Check sheet for the modelled part. Datum: model origin and axes. Units: mm. Round coordinates to 2 decimals unless told otherwise and drop trailing zeros. Loops run counter-clockwise (first coordinate to the right, second up) from the corner with the lowest first, then second, coordinate; pieces in that order, holes last. Notation, with made-up numbers: M 10.25,50 L 37.25,50 A17 cw 37.25,73 Z; hole C 73.25,8.25 d2. An arc over 180 degrees is marked long. One line per question, with ' | ' between items. Start each with the question number.
(1) Draft check along Y on faces 1 (the face through (55.076, 154.307, -0.986)), 2 (the face through (27, 58, 0)). Enter one of: +Y half, -Y half, draft (parallel to the pull), parting line (faces both ways), or undercut.
(2) Section check A-A (x = -23). Record the boundary of the cut face in (y, z), and give its area (3 significant figures).
(3) Section check C-C (y = 34). Record the boundary of the cut face in (x, z), and give its area (3 significant figures).
(4) Thickness scan on probe 1 along X at (y, z) = (214.3, -1.4); probe 2 along X at (y, z) = (191.85, -0.95); probe 3 along Y at (x, z) = (-31.35, -1.35). Record the ranges inside material, lowest first. Write a range as [from, to].
(5) Section check B-B (z = -0.85). Count the separate pieces of the cut face and the enclosed holes in it, and give its area (3 significant figures).
(6) Go/stop test with a flat-tipped pin: P1, Ø2, axis at x = 16.5, y = 27, coming from the +Z side. Record where the tip stops, or that it passes through.
```python
from build123d import *

# Parameters (mm, degrees)
SKETCH1_R           = 1.6
SKETCH1_R_2         = 20
SKETCH1_R_3         = 1.25
BOSS_EXTRUDE1_DEPTH = 2


with BuildPart() as part:
    # Sketch1 → Boss-Extrude1 (new body)
    with BuildSketch(Plane(origin=(0, 0, 0), x_dir=(0, 1, 0), z_dir=(0, 0, 1))):
        Polygon((-98, 35), (-98, -90), (219.3, -90), (219.3, 35), (106.85, 35), (106.85, 6.35), (-57.15, 6.35), (-57.15, 35), align=None)
        with Locations(Location((205.3, 7.8, 0), (0, 0, 270))):
            Circle(SKETCH1_R, mode=Mode.SUBTRACT)
        with Locations(Location((-92.5, 8, 0), (0, 0, 270))):
            Circle(SKETCH1_R, mode=Mode.SUBTRACT)
        with Locations(Location((-93, 28, 0), (0, 0, 270))):
            Circle(SKETCH1_R, mode=Mode.SUBTRACT)
        with Locations(Location((114.3, 0, 0), (0, 0, 270))):
            Circle(SKETCH1_R, mode=Mode.SUBTRACT)
        with Locations(Location((-93, -83, 0), (0, 0, 270))):
            Circle(SKETCH1_R, mode=Mode.SUBTRACT)
        with Locations(Location((-86.5, -73, 0), (0, 0, 270))):
            Circle(SKETCH1_R, mode=Mode.SUBTRACT)
        with Locations(Location((64.3, -83, 0), (0, 0, 270))):
            Circle(SKETCH1_R, mode=Mode.SUBTRACT)
        with Locations(Location((75.7, -78, 0), (0, 0, 270))):
            Circle(SKETCH1_R, mode=Mode.SUBTRACT)
        with Locations(Location((214.3, -83, 0), (0, 0, 270))):
            Circle(SKETCH1_R, mode=Mode.SUBTRACT)
        with Locations(Location((208.3, -65, 0), (0, 0, 270))):
            Circle(SKETCH1_R, mode=Mode.SUBTRACT)
        with Locations(Location((181.3, -56, 0), (0, 0, 270))):
            Circle(SKETCH1_R, mode=Mode.SUBTRACT)
        with Locations(Location((148.3, -36, 0), (0, 0, 270))):
            Circle(SKETCH1_R_2, mode=Mode.SUBTRACT)
        with Locations(Location((0, 0, 0), (0, 0, 270))):
            Circle(SKETCH1_R, mode=Mode.SUBTRACT)
        with Locations(Location((104.8, -18, 0), (0, 0, 270))):
            Circle(SKETCH1_R, mode=Mode.SUBTRACT)
        with Locations(Location((191.85, 31.35, 0), (0, 0, 270))):
            Circle(SKETCH1_R_3, mode=Mode.SUBTRACT)
        with Locations(Location((121.85, 11.35, 0), (0, 0, 270))):
            Circle(SKETCH1_R_3, mode=Mode.SUBTRACT)
        with Locations(Location((111.3, 28, 0), (0, 0, 270))):
            Circle(SKETCH1_R, mode=Mode.SUBTRACT)
        with Locations(Location((121.85, 31.35, 0), (0, 0, 270))):
            Circle(SKETCH1_R_3, mode=Mode.SUBTRACT)
        with Locations(Location((191.85, 11.35, 0), (0, 0, 270))):
            Circle(SKETCH1_R_3, mode=Mode.SUBTRACT)
        with Locations(Location((214.3, 28, 0), (0, 0, 270))):
            Circle(SKETCH1_R, mode=Mode.SUBTRACT)
    extrude(amount=-BOSS_EXTRUDE1_DEPTH)


solid = part.part
```
The answers:
1) face 1: undercut | face 2: draft
2) outline: M -98,-2 L -57.15,-2 L -57.15,0 L -98,0 Z; M 106.85,-2 L 219.3,-2 L 219.3,0 L 106.85,0 Z | area: 307 mm²
3) outline: M -6.35,-2 L 90,-2 L 90,0 L -6.35,0 Z | area: 193 mm²
4) probe 1: [-35, -29.6], [-26.4, 81.4], [84.6, 90] | probe 2: [-35, -32.6], [-30.1, -12.6], [-10.1, 90] | probe 3: [-98, -57.15], [106.85, 120.6], [123.1, 190.6], [193.1, 219.3]
5) separate pieces: 1 | enclosed holes: 20 | area: 33,600 mm²
6) P1: z = 0
